Could you check a few things on this model? Use its own coordinates, in mm. A direction names the side the tool comes from. Round coordinates to 2 decimals unless told otherwise and drop trailing zeros. Write each loop counter-clockwise with the first axis right and the second up, starting at its lowest first coordinate (ties: lowest second). Pieces come first, ordered by that corner, then holes. Notation, with made-up numbers: (-3, 55.25) - (47, 55.25) arc R25 ccw to (47, 76.25) - close; hole circle Ø8 at (45, -16). An arc over 180 degrees is marked (long way). Write each question's results on one line, items separated by ' | '. Start each with the question number.
(1) Imagine slicing it at C-C on z = -35.25. Write out the boundary of the cut face in (x, y).
(2) Thinking about a two-plate mould opening in Z: for faces 6 (the cylindrical face through (37.042, -81.056, -25.112)), 7 (the cylindrical face through (17.14, -78.13, -41.49)), 8 (the cylindrical face through (-20.14, 13.01, -58.1)), 9 (the flat face through (-30, 21, -35)), which applies, +Z half, -Z half, draft (parallel to the pull), parting line (faces both ways), or undercut?
(3) On a 3-axis mill with a long thin cutter (end or side, diameter ignored), from which of +Z, -Z, +X, -X, +Y, -Y can I reach the whole of each face in a straight line? I mean faces 1 (the flat face through (-5, -10, -35)), 2 (the flat face through (-10, 34, -36)), 3 (the flat face through (0, 0, -70.5)), 4 (the flat face through (34, -60, -32)), 5 (the flat face through (20, -27, -35)). Say none if no direction works.
(4) For P1, Ø6, axis at y = -5.5, z = -58.5, coming from the +X side; P2, Ø6, axis at x = -18.5, y = 36.5, coming from the -Z side; P3, Ø3, axis at x = 32.5, z = -45, coming from the +Y side, each with a flat end and sliding along its axis, tell me the tip position at first contact or that it passes through.
(5) Imagine slicing it at A-A on x = 7. Write out the boundary of the cut face in (y, z), then the cut area to 3 significant figures.
(6) Imagine slicing it at D-D on x = -13.5. Write out the boundary of the cut face in (y, z), then the cut area to 3 significant figures.
(7) Imagine slicing it at B-B on y = -76.5. Write out the boundary of the cut face in (x, z).
(8) Please list where these lines run through material, in increasing order: line 1 (Z direction, x = 14.5, y = -70); line 2 (Y direction, x = 18.5, z = -39.5); line 3 (Z direction, x = -24.5, y = 50). Write a range as [from, to].
```python
from build123d import *

# Parameters (mm, degrees)
BOSS_EXTRUDE1_DEPTH      = 70.5
BOSS_EXTRUDE2_DEPTH      = 10
BOSS_EXTRUDE2_DEPTH_BACK = 30.2
SKETCH2_R                = 30
SKETCH3_R                = 10.25
CUT_EXTRUDE1_DEPTH       = 92
SKETCH4_R                = 15
CUT_EXTRUDE2_DEPTH       = 6
CUT_EXTRUDE_THIN1_DEPTH  = 53
SKETCH7_R                = 7.5
BOSS_EXTRUDE5_DEPTH      = 20


with BuildPart() as part:
    # Sketch1 → Boss-Extrude1 (new body)
    with BuildSketch(Plane.XY):
        Polygon((-30, 10), (30, 10), (30, -70), (20, -70), (20, -10), (-30, -10), align=None)
    extrude(amount=-BOSS_EXTRUDE1_DEPTH)

    # Sketch2 → Boss-Extrude2 (add, two sides: drawn at the far end of the back side and taken through both)
    with BuildSketch(Plane(origin=(30, 0, 0), x_dir=(0, 0, -1), z_dir=(1, 0, 0)).offset(-BOSS_EXTRUDE2_DEPTH_BACK)):
        with Locations(Location((35.25, -70, 0), (0, 0, 90))):
            Circle(SKETCH2_R)
    extrude(amount=BOSS_EXTRUDE2_DEPTH + BOSS_EXTRUDE2_DEPTH_BACK)

    # Sketch3 → Cut-Extrude1 (cut)
    with BuildSketch(Plane(origin=(40, 0, 0), x_dir=(0, 0, -1), z_dir=(1, 0, 0))):
        with Locations(Location((35.25, -70, 0), (0, 0, 90))):
            Circle(SKETCH3_R)
    extrude(amount=-CUT_EXTRUDE1_DEPTH, mode=Mode.SUBTRACT)

    # Sketch4 → Cut-Extrude2 (cut)
    with BuildSketch(Plane(origin=(40, 0, 0), x_dir=(0, 0, -1), z_dir=(1, 0, 0))):
        with Locations(Location((35.25, -70, 0), (0, 0, 90))):
            Circle(SKETCH4_R)
    extrude(amount=-CUT_EXTRUDE2_DEPTH, mode=Mode.SUBTRACT)

    # Sketch5 → Cut-Extrude-Thin1 (cut)
    with BuildSketch(Plane(origin=(30, 0, 0), x_dir=(0, 0, -1), z_dir=(1, 0, 0))):
        Polygon((0, -10), (5.25, -70), (-4.711937175, -70.871669503), (-9.961937175, -10.871669503), align=None)
        Polygon((65.25, -70), (70.5, -10), (80.461937175, -10.871669503), (75.211937175, -70.871669503), align=None)
    extrude(amount=-CUT_EXTRUDE_THIN1_DEPTH, mode=Mode.SUBTRACT)

    # Sketch7 → Boss-Extrude5 (add)
    with BuildSketch(Plane.ZY.offset(30)):
        with BuildLine():
            ThreePointArc((-15.25, 50), (-35.25, 70), (-55.25, 50))
            Line((-55.25, 50), (-55.25, 20))
            ThreePointArc((-55.25, 20), (-58.178932188, 12.928932188), (-65.25, 10))
            Line((-65.25, 10), (-5.25, 10))
            ThreePointArc((-5.25, 10), (-12.321067812, 12.928932188), (-15.25, 20))
            Line((-15.25, 20), (-15.25, 50))
        make_face()
        with Locations(Location((-35.25, 50, 0), (0, 0, 270))):
            Circle(SKETCH7_R, mode=Mode.SUBTRACT)
    extrude(amount=-BOSS_EXTRUDE5_DEPTH)


solid = part.part
```
Response:
1) outline: (-30, -10) - (20, -10) - (20, -40) - (-0.2, -40) - (-0.2, -59.75) - (34, -59.75) - (34, -55) - (40, -55) - (40, -40) - (30, -40) - (30, 10) - (-10, 10) - (-10, 42.5) - (-30, 42.5) - close; (-30, 57.5) - (-10, 57.5) - (-10, 70) - (-30, 70) - close; (-0.2, -100) - (40, -100) - (40, -85) - (34, -85) - (34, -80.25) - (-0.2, -80.25) - close
2) face 6: undercut | face 7: undercut | face 8: -Z half | face 9: draft
3) face 1: +Z, -Z, -X | face 2: +Z, -Z, +X, +Y | face 3: -Z, +X, -X, +Y, -Y | face 4: +X | face 5: -X
4) P1: x = 30 | P2: z = -55.25 | P3: y = -41.16
5) outline: circle Ø60 at (-70, -35.25); (-10, -70.5) - (10, -70.5) - (10, 0) - (-10, 0) - close; hole circle Ø20.5 at (-70, -35.25) | area: 3,910 mm²
6) outline: (-10, -70.5) - (10, -70.5) - (10, -65.25) arc R10 cw to (20, -55.25) - (50, -55.25) arc R20 ccw to (50, -15.25) - (20, -15.25) arc R10 cw to (10, -5.25) - (10, 0) - (-10, 0) - close; hole circle Ø15 at (50, -35.25) | area: 3,500 mm²
7) outline: (-0.2, -64.54) - (40, -64.54) - (40, -48.77) - (34, -48.77) - (34, -43.18) - (-0.2, -43.18) - close; (-0.2, -27.32) - (34, -27.32) - (34, -21.73) - (40, -21.73) - (40, -5.96) - (-0.2, -5.96) - close
8) line 1: [-65.25, -45.5], [-25, -5.25] | line 2: [-99.7, -79.33], [-60.67, -40.3], [-10, 10] | line 3: [-55.25, -42.75], [-27.75, -15.25]
